Can you work these out from the drawing? Everything is in mm from the part's minimum corner. A direction names the side the tool comes from. Coordinates: 2 decimals unless noted, no trailing zeros. Write each loop counter-clockwise with the first axis right and the second up, starting at its lowest first coordinate (ties: lowest second). Pieces come first, ordered by that corner, then holes.
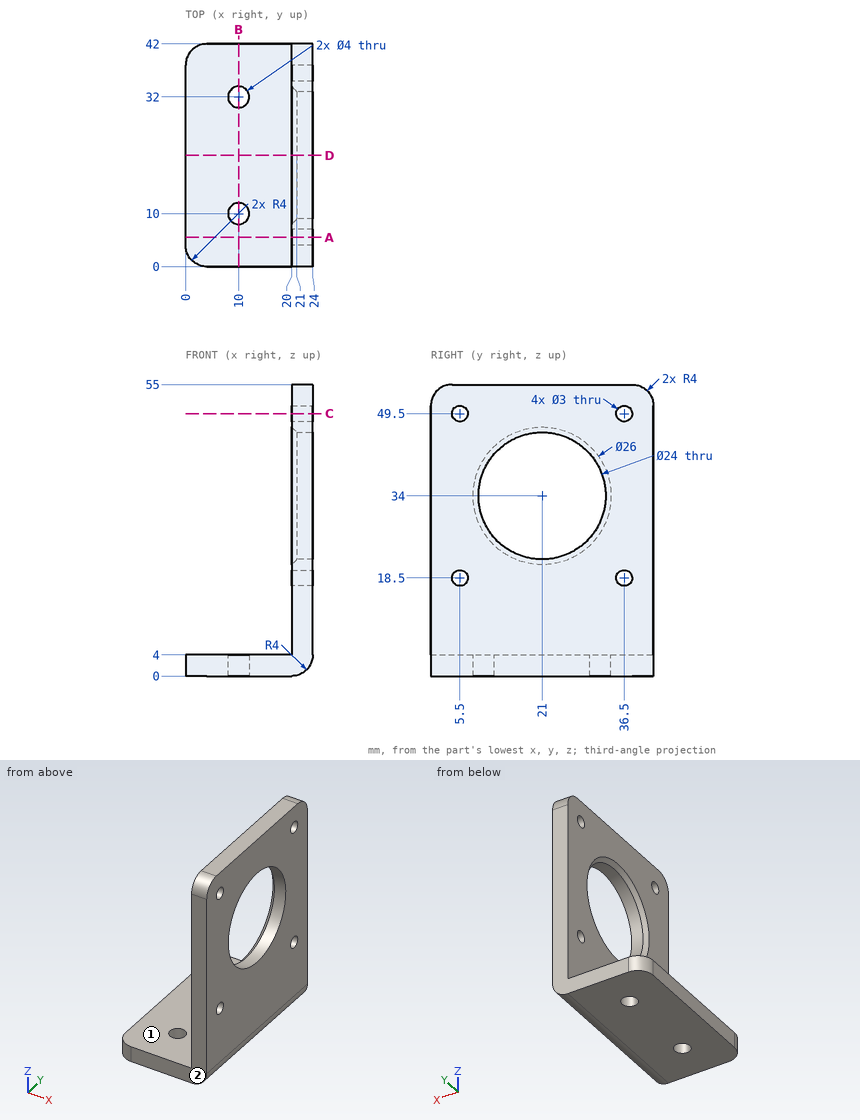
1. I want a section at A-A (y = 5.5). List the corners of the cut face in (x, z) for me.
2. I want a section at B-B (x = 10). List the corners of the cut face in (y, z) for me.
3. I want a section at D-D (y = 21). List the corners of the cut face in (x, z) for me.
4. I want a section at C-C (z = 49.5). List the corners of the cut face in (x, y) for me, then the cut area to 3 significant figures.
5. On a 3-axis mill with a long thin cutter (end or side, diameter ignored), from which of +Z, -Z, +X, -X, +Y, -Y can I reach the whole of each face in a straight line? I mean the marked faces 1 and 2. Say none if no direction works.
6. If I drill on line 1 (Y direction, x = 10, z = 2.4); line 2 (Y direction, x = 22.75, z = 49.5); line 3 (Z direction, x = 10.5, y = 34), over which ranges is the centre line in solid material (lowest first)?
7. For pin 1 Ø4.5 at (x, y) = (10, 32) entering from +Z; pin 2 Ø5 at (y, z) = (5.5, 18.5) entering from -X, each with a flat end and sliding along its axis, tell me the tip position at first contact or that it passes through.
Response values:
1. outline: (0, 0) - (20, 0) arc R4 ccw to (24, 4) - (24, 17) - (20, 17) - (20, 4) - (0, 4) - close; (20, 20) - (24, 20) - (24, 48) - (20, 48) - close; (20, 51) - (24, 51) - (24, 55) - (20, 55) - close
2. outline: (0, 0) - (8, 0) - (8, 4) - (0, 4) - close; (12, 0) - (30, 0) - (30, 4) - (12, 4) - close; (34, 0) - (42, 0) - (42, 4) - (34, 4) - close
3. outline: (0, 0) - (20, 0) arc R4 ccw to (24, 4) - (24, 22) - (21, 22) - (20, 21) - (20, 4) - (0, 4) - close; (20, 47) - (21, 46) - (24, 46) - (24, 55) - (20, 55) - close
4. outline: (20, 0) - (24, 0) - (24, 4) - (20, 4) - close; (20, 7) - (24, 7) - (24, 35) - (20, 35) - close; (20, 38) - (24, 38) - (24, 42) - (20, 42) - close
4. area: 144 mm2
5. face 1: +Z, -X, +Y, -Y
5. face 2: +Z, -Z, +X, -X, -Y
6. line 1: y = 0 to 8, 12 to 30, 34 to 42
6. line 2: y = 0 to 4, 7 to 35, 38 to 42
6. line 3: z = 0 to 4
7. pin 1: stops at z = 4
7. pin 2: stops at x = 20
